The figure shows three views and two pictorial views of one solid part (mm, origin at its lowest corner). Answer the questions. A direction names the side the tool comes from. Coordinates: 2 decimals unless noted, no trailing zeros. Order: outer loops, then holes, each group sorted by start corner. A loop starts at its lowest first (then second) coordinate and runs counter-clockwise, first axis right, second up. Notation, with made-up numbers: (80, 87) -> (117, 87) arc R22 cw to (117, 115) -> close; hole circle Ø9 at (-22, 75). An arc over 180 degrees is marked (long way). Write item = value, one per line.
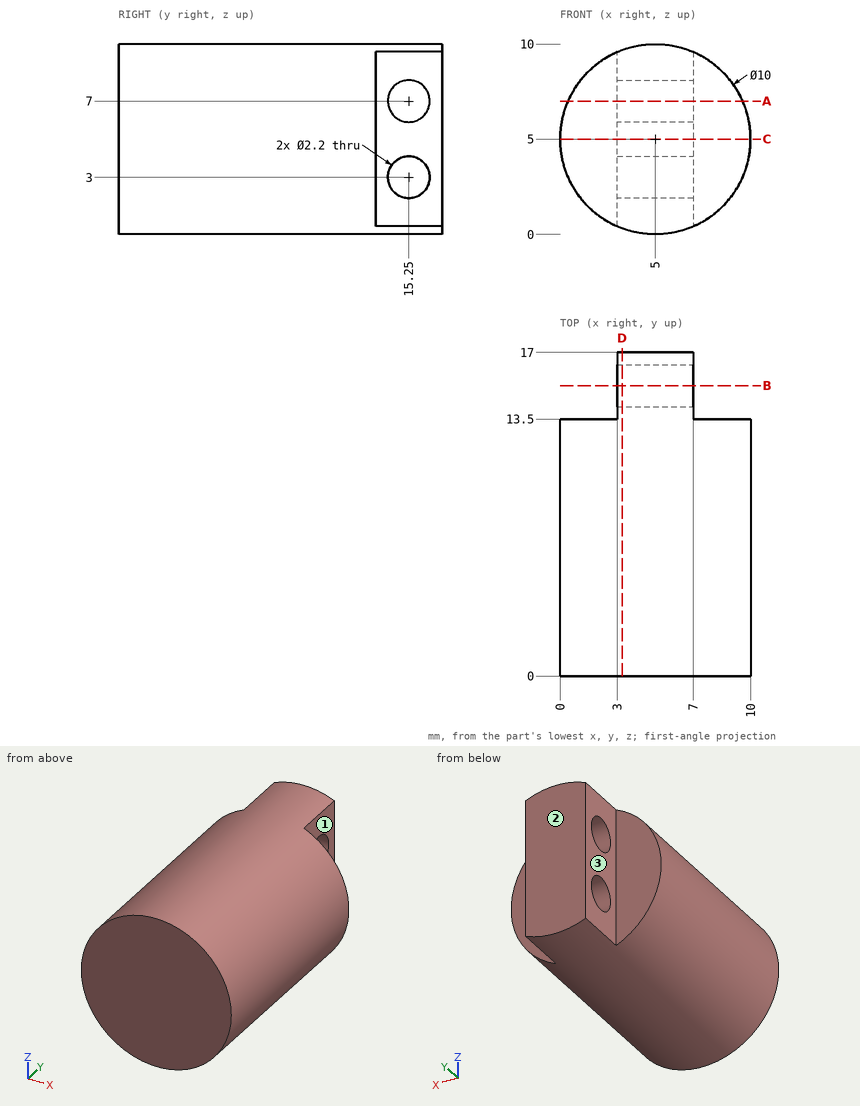
Q1. Section D-D, the plane x = 3.25 is taken. Give the vertices of the cut face in (y, z), plus the area to 3 significant figures.
The answers:
outline = (0, 0.32) -> (17, 0.32) -> (17, 9.68) -> (0, 9.68) -> close; hole circle Ø2.2 at (15.25, 3); hole circle Ø2.2 at (15.25, 7)
area = 152 mm2
Q2. Section A-A, the plane z = 7 is taken. Give the vertices of the cut face in (x, y), plus the area to 3 significant figures.
The answers:
outline = (0.42, 0) -> (9.58, 0) -> (9.58, 13.5) -> (7, 13.5) -> (7, 14.15) -> (3, 14.15) -> (3, 13.5) -> (0.42, 13.5) -> close; (3, 16.35) -> (7, 16.35) -> (7, 17) -> (3, 17) -> close
area = 129 mm2
Q3. Section B-B, the plane y = 15.25 is taken. Give the vertices of the cut face in (x, z), plus the area to 3 significant figures.
The answers:
outline = (3, 0.42) arc R5 ccw to (7, 0.42) -> (7, 1.9) -> (3, 1.9) -> close; (3, 4.1) -> (7, 4.1) -> (7, 5.9) -> (3, 5.9) -> close; (3, 8.1) -> (7, 8.1) -> (7, 9.58) arc R5 ccw to (3, 9.58) -> close
area = 21.3 mm2
Q4. Find the intervals of material crossed by line 1 along Y through (x, z) = (4.25, 3); line 2 along X through (y, z) = (13.75, 6); line 3 along Y through (x, z) = (8.5, 6.25), in increasing order.
The answers:
line_1 = 0 to 14.15, 16.35 to 17
line_2 = 3 to 7
line_3 = 0 to 13.5
Q5. Each of these flat-tipped pins is pushed along its axis until it touches: pin 1 Ø2 at (x, y) = (3, 7.5) entering from -Z; pin 2 Ø2.5 at (x, z) = (1.5, 5.5) entering from +Y; pin 3 Ø4 at (x, y) = (8.5, 2) entering from +Z; pin 4 Ø1.8 at (y, z) = (15.25, 7) entering from -X. Where does it stop, or does it pass through?
The answers:
pin_1 = 0.1
pin_2 = 13.5
pin_3 = 9.77
pin_4 = through
Q6. Section C-C, the plane z = 5 is taken. Give the vertices of the cut face in (x, y), plus the area to 3 significant figures.
The answers:
outline = (0, 0) -> (10, 0) -> (10, 13.5) -> (7, 13.5) -> (7, 17) -> (3, 17) -> (3, 13.5) -> (0, 13.5) -> close
area = 149 mm2
Q7. A tool of negligible diameter and unlimited length cuts with its end or side. For the marked faces 1, 2 and 3, from which of +Z, -Z, +X, -X, +Y, -Y can it reach the whole face along a straight path? Write none if from no direction.
The answers:
face_1 = +Z, -Z, +X, +Y
face_2 = +Z, -Z, +X, -X, +Y
face_3 = +Z, -Z, -X, +Y
